```python
from build123d import *

# Parameters (mm, degrees)
BOX_W        = 60
BOX_H        = 17
BOX_DEPTH    = 17
FILLET001_R  = 1
FILLET002_R  = 0.5
BOX008_W     = 89
BOX008_H     = 15
BOX008_DEPTH = 2
FILLET003_R  = 0.25


with BuildPart() as obj1:
    # Box → Box (new body)
    with BuildSketch(Plane(origin=(0, -8.5, -17), x_dir=(1, 0, 0), z_dir=(0, 0, 1))):
        with Locations((30, 8.5)):
            Rectangle(BOX_W, BOX_H)
    extrude(amount=BOX_DEPTH)

    # Fillet001
    fillet001_edges = [obj1.edges().sort_by_distance(p)[0] for p in [
        (0, -8.5, -8.5),
        (0, 8.5, -8.5),
        (60, -8.5, -8.5),
        (60, 8.5, -8.5),
    ]]
    fillet(fillet001_edges, radius=FILLET001_R)

    # Fillet002
    fillet002_edges = [obj1.edges().sort_by_distance(p)[0] for p in [
        (0, 0, 0),
        (0, 0, -17),
        (30, -8.5, 0),
        (30, 8.5, 0),
        (60, 0, 0),
        (30, -8.5, -17),
        (30, 8.5, -17),
        (60, 0, -17),
    ]]
    fillet(fillet002_edges, radius=FILLET002_R)


with BuildPart() as obj1_1:
    # Fillet002 placement: moved
    add(obj1.part.moved(Location((35, 0, -2.5))))


with BuildPart() as fusion035:
    # Box008 → Box008 (new body)
    with BuildSketch(Plane(origin=(0, -6.5, -2), x_dir=(1, 0, 0), z_dir=(0, 0, 1))):
        with Locations((44.5, 7.5)):
            Rectangle(BOX008_W, BOX008_H)
    extrude(amount=BOX008_DEPTH)

    # Fillet003
    fillet003_edges = [fusion035.edges().sort_by_distance(p)[0] for p in [
        (0, -6.5, -1),
        (0, 1, 0),
        (0, 8.5, -1),
        (0, 1, -2),
        (89, -6.5, -1),
        (89, 1, 0),
        (89, 8.5, -1),
        (89, 1, -2),
        (44.5, -6.5, -2),
        (44.5, -6.5, 0),
        (44.5, 8.5, -2),
        (44.5, 8.5, 0),
    ]]
    fillet(fillet003_edges, radius=FILLET003_R)


with BuildPart() as fusion035_1:
    # Fillet003 placement: moved
    add(fusion035.part.moved(Location((20, 0, -19.5))))

    # Fusion035: union obj1
    add(obj1_1.part)


solid = fusion035_1.part
```
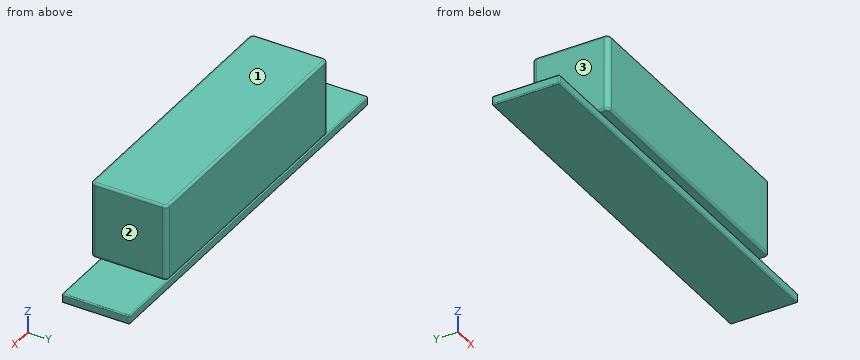
Input: part model. Units: mm. Frame: model coordinates. Face numbers are marked on the shaded views. A direction names the side the tool comes from. Give positions to 0.01 mm unless a question says otherwise; leave off trailing zeros. Order: outer loops, then holes, each group sorted by start corner. A loop starts at its lowest first (then second) coordinate and runs counter-clockwise, first axis right, second up.
1. Section A-A on z = -5.5. Return the cut outline in (x, y), and give its area (3 significant figures).
Derived:
outline: (35, -7.5) arc R1 ccw to (36, -8.5) - (94, -8.5) arc R1 ccw to (95, -7.5) - (95, 7.5) arc R1 ccw to (94, 8.5) - (36, 8.5) arc R1 ccw to (35, 7.5) - close
area: 1,020 mm2
2. Section B-B on y = -5.5. Return the cut outline in (x, z).
Derived:
outline: (20, -21.25) arc R0.25 ccw to (20.25, -21.5) - (108.75, -21.5) arc R0.25 ccw to (109, -21.25) - (109, -19.75) arc R0.25 ccw to (108.75, -19.5) - (94.5, -19.5) arc R0.5 ccw to (95, -19) - (95, -3) arc R0.5 ccw to (94.5, -2.5) - (35.5, -2.5) arc R0.5 ccw to (35, -3) - (35, -19) arc R0.5 ccw to (35.5, -19.5) - (20.25, -19.5) arc R0.25 ccw to (20, -19.75) - close
3. Reachability of the marked faces 1, 2 and 3 from +Z, -Z, +X, -X, +Y, -Y: full face, straight path, thin tool, end or side. Return the list, or none.
Derived:
face 1: +Z, +X, -X, +Y, -Y
face 2: +Z, +X, +Y, -Y
face 3: +Z, -X, +Y, -Y
4. Material intervals for L1, parallel to X at y = -7.5, z = -12.75; L2, parallel to Z at x = 34, y = -3; L3, parallel to Y at x = 91.5, z = -20.5, sorted ascending.
Derived:
L1: x = 35 to 95
L2: z = -21.5 to -19.5
L3: y = -6.5 to 8.5
5. Pin query (flat end, axial travel): pin 1 (0.8 mm diameter, centred on x = 47, z = -20.5, fed in from -Y); pin 2 (1.5 mm diameter, centred on y = 3.5, z = -10.5, fed in from -X); pin 3 (7.5 mm diameter, centred on y = 1, z = -14, fed in from +X). Return the tip coordinate at first contact, or that it passes through.
Derived:
pin 1: stops at y = -6.5
pin 2: stops at x = 35
pin 3: stops at x = 95
